Here's how the part is built. I have some questions about the finished solid (model axes, mm). Face numbers are marked on the shaded views. A direction names the side the tool comes from. Coordinates: 2 decimals unless noted, no trailing zeros. Loops run counter-clockwise (first coordinate to the right, second up) from the corner with the lowest first, then second, coordinate; pieces in that order, holes last. Notation, with made-up numbers: M -30,44 L -11,44 A23 ccw -11,65 Z; hole C 60,-13.5 d9. An arc over 180 degrees is marked long. Use one line per item in the form item = value. Start each with the question number.
(1) Will these pins go through, and if not, where does the flat tip stop? P1, Ø1, axis at x = 4, z = -24, coming from the -Y side; P2, Ø5, axis at y = 46.5, z = -9, coming from the -X side; P3, Ø1, axis at x = 1, z = -26.5, coming from the +Y side.
(2) Thinking about a two-plate mould opening in Y: for the marked faces 3, 4, 5 and 6, which applies, +Y half, -Y half, draft (parallel to the pull), parting line (faces both ways), or undercut?
(3) On a 3-axis mill with a long thin cutter (end or side, diameter ignored), from which of +Z, -Z, +X, -X, +Y, -Y can I reach the whole of each face in a straight line? I mean the marked faces 1 and 2. Say none if no direction works.
(4) Imagine slicing it at C-C, the plane y = 60. Please give me the cut outline in (x, z), and give its area (3 significant figures).
(5) Imagine slicing it at A-A, the plane z = -20.32. Please give me the cut outline in (x, y), and give its area (3 significant figures).
(6) Please list where these lines run through material, in increasing order: L1, parallel to Z at x = 5.25, y = 4; L2, parallel to Y at x = 3.25, z = -20.32; L3, parallel to Y at x = 4.5, z = -14.5.
(7) Imagine slicing it at B-B, the plane x = 5. Please give me the cut outline in (y, z).
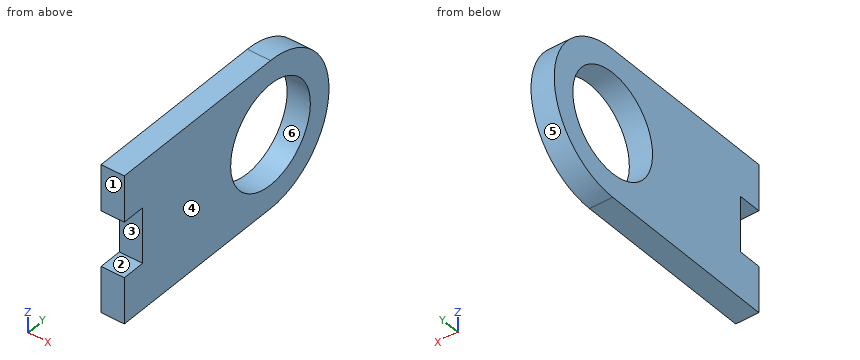
```python
from build123d import *

# Parameters (mm, degrees)
SKETCH1_R           = 13.85
BOSS_EXTRUDE1_DEPTH = 6.35


with BuildPart() as part:
    # Sketch1 → Boss-Extrude1 (new body)
    with BuildSketch(Plane(origin=(0, 0, 0), x_dir=(0, 0, -1), z_dir=(1, 0, 0))):
        with BuildLine():
            Line((27.94, 0), (40.64, 0))
            Line((40.64, 0), (40.64, 50.8))
            ThreePointArc((40.64, 50.8), (20.32, 71.12), (0, 50.8))
            Line((0, 50.8), (0, 0))
            Line((0, 0), (12.7, 0))
            Line((12.7, 0), (12.7, 6.35))
            Line((12.7, 6.35), (27.94, 6.35))
            Line((27.94, 6.35), (27.94, 0))
        make_face()
        with Locations((20.32, 50.8)):
            Circle(SKETCH1_R, mode=Mode.SUBTRACT)
    extrude(amount=BOSS_EXTRUDE1_DEPTH)


solid = part.part
```
Answer:
q1.P1 = 6.35
q1.P2 = 0
q1.P3 = 70.31
q2.face_3 = -Y half
q2.face_4 = draft
q2.face_5 = +Y half
q2.face_6 = undercut
q3.face_1 = +Z, -Z, +X, -X, -Y
q3.face_2 = +X, -X, -Y
q4.outline = M 0,-38.44 L 6.35,-38.44 L 6.35,-30.67 L 0,-30.67 Z; M 0,-9.97 L 6.35,-9.97 L 6.35,-2.2 L 0,-2.2 Z
q4.area = 98.6 mm²
q5.outline = M 0,6.35 L 6.35,6.35 L 6.35,36.95 L 0,36.95 Z; M 0,64.65 L 6.35,64.65 L 6.35,71.12 L 0,71.12 Z
q5.area = 235 mm²
q6.L1 = -40.64 to -27.94, -12.7 to 0
q6.L2 = 6.35 to 36.95, 64.65 to 71.12
q6.L3 = 6.35 to 38.23, 63.37 to 70.27
q7.outline = M 0,-40.64 L 50.8,-40.64 A20.32 ccw 50.8,0 L 0,0 L 0,-12.7 L 6.35,-12.7 L 6.35,-27.94 L 0,-27.94 Z; hole C 50.8,-20.32 d27.7
